CAD build for the part. Positions are in the model's coordinates, mm. Face numbers are marked on the shaded views. A direction names the side the tool comes from. Round coordinates to 2 decimals unless told otherwise and drop trailing zeros. Write each loop counter-clockwise with the first axis right and the second up, starting at its lowest first coordinate (ties: lowest second). Pieces come first, ordered by that corner, then holes. Notation, with made-up numbers: (20.25, 49) - (68.25, 49) arc R10 ccw to (68.25, 64) - close; hole circle Ø2 at (19.25, 20). An arc over 180 degrees is marked (long way). Put each result on its own line as item: value. Start each with the question number.
Item 1: Cut at C-C (x = 0). Give the cut face in (y, z), and give its area (3 significant figures).
Item 2: Cut at B-B (y = 0). Give the cut face in (x, z), and give its area (3 significant figures).
Item 3: Cut at D-D (z = 45). Give the cut face in (x, y), and give its area (3 significant figures).
Item 4: Drill centre lines: line 1 (X direction, y = -4, z = 11.5); line 2 (Y direction, x = 0, z = 3.45); line 3 (Z direction, x = 9.5, y = -18.5). Where is each one in solid material? Low to high. Write a range as from..to.
Item 5: 3-axis set-ups, long thin cutter, end or side, ignore diameter. For the marked faces 1 and 2: which of +Z, -Z, +X, -X, +Y, -Y reach the whole face in a straight line?
Item 6: Pin check, flat tips, straight feed: pin 1 Ø15 at (y, z) = (-0.5, 38.5) entering from -X; pin 2 Ø12 at (y, z) = (0, 45) entering from -X; pin 3 Ø1 at (x, y) = (-2.5, -13.5) entering from +Z. Stop position of each tip, or through.
Item 7: Mould opens along X. For the marked faces 3, 4, 5 and 6 say: released by +X, released by -X, zero draft, split by the parting line, or undercut.
Item 8: Cut at A-A (z = 14). Give the cut face in (x, y).
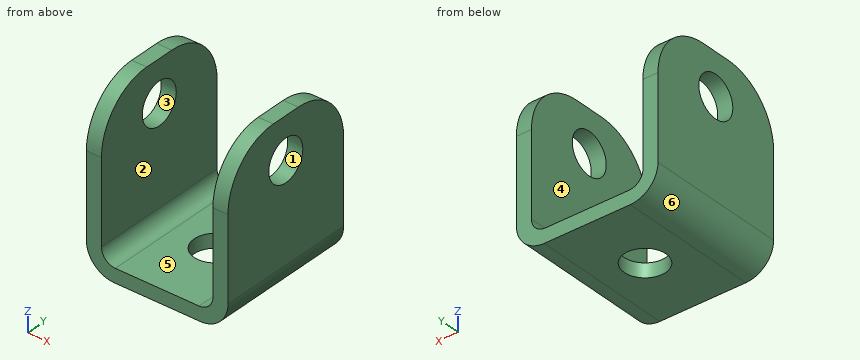
```python
from build123d import *

# Parameters (mm, degrees)
F0_W          = 51
F0_H          = 51
F1_DEPTH      = 60
F2_W          = 40.138214
F2_H          = 55
F3_DEPTH      = 51
F4_R          = 7.5
F5_DEPTH      = 60.001
F6_R          = 7.5
F7_DEPTH      = 25.501
F7_DEPTH_BACK = 88.263765
F8_R          = 10
F9_R          = 5
F10_R         = 20


with BuildPart() as f1:
    # F0 (on Top) → F1 (new body)
    with BuildSketch(Plane.XY):
        Rectangle(F0_W, F0_H)
    extrude(amount=F1_DEPTH)

    # F2 (on face) → F3 (cut)
    with BuildSketch(Plane.XZ.offset(25.5)):
        with Locations((0, 32.5)):
            Rectangle(F2_W, F2_H)
    extrude(amount=-F3_DEPTH, mode=Mode.SUBTRACT)

    # F4 (on Top) → F5 (cut, through all)
    with BuildSketch(Plane.XY):
        Circle(F4_R)
    extrude(amount=F5_DEPTH, mode=Mode.SUBTRACT)

    # F6 (on Right) → F7 (cut, two sides)
    with BuildSketch(Plane.YZ) as f7_sk:
        with Locations((0, 45)):
            Circle(F6_R)
    extrude(amount=F7_DEPTH, mode=Mode.SUBTRACT)
    extrude(f7_sk.sketch, amount=-F7_DEPTH_BACK, mode=Mode.SUBTRACT)

    # F8
    f8_edges = [f1.edges().sort_by_distance(p)[0] for p in [
        (-25.5, 0, 0),
        (25.5, 0, 0),
    ]]
    fillet(f8_edges, radius=F8_R)

    # F9
    f9_edges = [f1.edges().sort_by_distance(p)[0] for p in [
        (-20.069107, 0, 5),
        (20.069107, 0, 5),
    ]]
    fillet(f9_edges, radius=F9_R)

    # F10
    f10_edges = [f1.edges().sort_by_distance(p)[0] for p in [
        (22.784554, 25.5, 60),
        (-22.784554, 25.5, 60),
        (22.784554, -25.5, 60),
        (-22.784554, -25.5, 60),
    ]]
    fillet(f10_edges, radius=F10_R)


solid = f1.part
```
Output values:
1. outline: (-25.5, 0) - (-7.5, 0) - (-7.5, 5) - (-25.5, 5) - close; (7.5, 0) - (25.5, 0) - (25.5, 5) - (7.5, 5) - close
1. area: 180 mm2
2. outline: (-25.5, 10) arc R10 ccw to (-15.5, 0) - (-7.5, 0) - (-7.5, 5) - (-15.07, 5) arc R5 cw to (-20.07, 10) - (-20.07, 37.5) - (-25.5, 37.5) - close; (-25.5, 52.5) - (-20.07, 52.5) - (-20.07, 60) - (-25.5, 60) - close; (7.5, 0) - (15.5, 0) arc R10 ccw to (25.5, 10) - (25.5, 37.5) - (20.07, 37.5) - (20.07, 10) arc R5 cw to (15.07, 5) - (7.5, 5) - close; (20.07, 52.5) - (25.5, 52.5) - (25.5, 60) - (20.07, 60) - close
2. area: 582 mm2
3. outline: (-25.5, -24.86) - (-20.07, -24.86) - (-20.07, -7.5) - (-25.5, -7.5) - close; (-25.5, 7.5) - (-20.07, 7.5) - (-20.07, 24.86) - (-25.5, 24.86) - close; (20.07, -24.86) - (25.5, -24.86) - (25.5, -7.5) - (20.07, -7.5) - close; (20.07, 7.5) - (25.5, 7.5) - (25.5, 24.86) - (20.07, 24.86) - close
3. area: 377 mm2
4. line 1: -25.5..-20.07, 20.07..25.5
4. line 2: -25.5..-7.5, 7.5..25.5
4. line 3: 0..5
5. face 1: +X, -X
5. face 2: +Z, +Y, -Y
6. pin 1: x = -25.5
6. pin 2: through
6. pin 3: z = 5
7. face 3: zero draft
7. face 4: undercut
7. face 5: undercut
7. face 6: released by -X
8. outline: (-25.5, -25.5) - (-20.07, -25.5) - (-20.07, 25.5) - (-25.5, 25.5) - close; (20.07, -25.5) - (25.5, -25.5) - (25.5, 25.5) - (20.07, 25.5) - close
